Read the model definition and answer for the solid it produces. Units are mm, in the model's axes. A direction names the side the tool comes from. Give positions to 0.01 mm unless a question says otherwise; leave off trailing zeros. Order: outer loops, then holes, each group sorted by start corner. A loop starts at its lowest first (then second) coordinate and runs counter-clockwise, first axis right, second up. Notation, with made-up numbers: (4, 22.25) - (12, 22.25) arc R18 cw to (12, 55.25) - close; hole circle Ø4 at (-18.75, 17). An arc over 180 degrees is marked (long way). One line per item, written item: value. Start each with the question number.
```python
from build123d import *

# Parameters (mm, degrees)
EXTRUDE_1_DEPTH     = 3
EXTRUDE_2_DEPTH     = 4
EXTRUDE_3_DEPTH     = 1
CHAMFER_1_SIZE      = 1
SKETCH_1_3_R        = 5.15
CUT_EXTRUDE_1_DEPTH = 5
FILLET_1_R          = 1.5
FILLET_2_R          = 1


with BuildPart() as part:
    # 草图1 → 凸台-拉伸1 (new body)
    with BuildSketch(Plane.XY):
        with BuildLine():
            Line((0, 15), (120, 15))
            ThreePointArc((120, 15), (135, 0), (120, -15))
            Line((120, -15), (0, -15))
            ThreePointArc((0, -15), (-15, 0), (0, 15))
        make_face()
    extrude(amount=EXTRUDE_1_DEPTH)

    # 草图2 → 凸台-拉伸2 (add)
    with BuildSketch(Plane.XY.offset(3)):
        with BuildLine():
            Line((-1.5, 4.769696007), (-1.5, -4.769696007))
            ThreePointArc((-1.5, -4.769696007), (-5, 0), (-1.5, 4.769696007))
        make_face()
        with BuildLine():
            Line((1.5, 4.769696007), (1.5, -4.769696007))
            ThreePointArc((1.5, -4.769696007), (5, 0), (1.5, 4.769696007))
        make_face()
    extrude(amount=EXTRUDE_2_DEPTH)

    # 草图5 → 凸台-拉伸3 (add)
    with BuildSketch(Plane.XY.offset(7)):
        with BuildLine():
            Line((-1.5, 5.291502622), (-1.5, -5.291502622))
            ThreePointArc((-1.5, -5.291502622), (-5.5, 0), (-1.5, 5.291502622))
        make_face()
        with BuildLine():
            Line((1.5, 5.291502622), (1.5, -5.291502622))
            ThreePointArc((1.5, -5.291502622), (5.5, 0), (1.5, 5.291502622))
        make_face()
    extrude(amount=EXTRUDE_3_DEPTH)

    # 倒角1
    chamfer_1_edges = [part.edges().sort_by_distance(p)[0] for p in [
        (5.5, 0, 8),
        (-5.5, 0, 8),
    ]]
    chamfer(chamfer_1_edges, length=CHAMFER_1_SIZE - 0.0001)  # a hair under: the kernel refuses the full size

    # 草图1<3> → 切除-拉伸1 (cut)
    with BuildSketch(Plane.XY):
        with Locations((120, 0)):
            Circle(SKETCH_1_3_R)
    extrude(amount=CUT_EXTRUDE_1_DEPTH, mode=Mode.SUBTRACT)

    # 圆角1
    fillet_1_edges = [part.edges().sort_by_distance(p)[0] for p in [
        (-1.5, 0, 3),
        (1.5, 0, 3),
    ]]
    fillet(fillet_1_edges, radius=FILLET_1_R - 0.0001)  # a hair under: the kernel refuses the full size

    # 圆角2
    fillet_2_edges = [part.edges().sort_by_distance(p)[0] for p in [
        (135, 0, 3),
        (60, 15, 3),
        (-15, 0, 3),
        (60, 15, 0),
        (135, 0, 0),
        (60, -15, 0),
        (-15, 0, 0),
        (60, -15, 3),
    ]]
    fillet(fillet_2_edges, radius=FILLET_2_R)


solid = part.part
```
1) For faces 4 (the flat face through (5.27, 0.02, 7)), 5 (the cylindrical face through (-5, 0, 5)), 6 (the flat face through (1.5, 0, 6)), determine the directions among +Z, -Z, +X, -X, +Y, -Y from which every point of the face is accessible in a straight line to the end or side of a thin tool.
2) Each of these flat-tipped pins is pushed along its axis until it touches: pin 1 (10 mm diameter, centred on x = 64.5, y = -3, fed in from +Z); pin 2 (4 mm diameter, centred on y = 1.5, z = 6, fed in from -X); pin 3 (1 mm diameter, centred on y = 5, z = 1, fed in from +X); pin 4 (2 mm diameter, centred on x = 77, z = 5, fed in from -Y). Where does it stop, or does it pass through?
3) Find the intervals of material crossed by probe 1 along X at (y, z) = (0, 2); probe 2 along Y at (x, z) = (120, 1.2); probe 3 along Z at (x, y) = (39, -10), in increasing order. Write a range as from..to.
4) Section B-B on x = 7 is taken. Write down the section's boundary in (y, z).
5) Section C-C on z = 5.75 is taken. Write down the section's boundary in (x, y), plus the area to 3 significant figures.
6) The mould has two halves that part along Z. Classify faces 1 (the cylindrical face through (134.996, 0.33, 1.493)), 2 (the flat face through (-3, 0, 8)), 3 (the flat face through (-5.27, 0.02, 7)): +Z half, -Z half, draft (parallel to the pull), parting line (faces both ways), or undercut.
Solved:
1. face 4: +X
1. face 5: -X
1. face 6: +Z, +Y, -Y
2. pin 1: stops at z = 3
2. pin 2: stops at x = -5.5
2. pin 3: stops at x = 134.31
2. pin 4: passes through
3. probe 1: x = -15..114.85, 125.15..135
3. probe 2: y = -15..-5.15, 5.15..15
3. probe 3: z = 0..3
4. outline: (-15, 1) arc R1 ccw to (-14, 0) - (14, 0) arc R1 ccw to (15, 1) - (15, 2) arc R1 ccw to (14, 3) - (-14, 3) arc R1 ccw to (-15, 2) - close
5. outline: (-1.5, -4.77) - (-1.5, 4.77) arc R5 ccw to start; (1.5, -4.77) arc R5 ccw to (1.5, 4.77) - close
5. area: 49.0 mm2
6. face 1: draft
6. face 2: +Z half
6. face 3: undercut
